Source: CAD feature listing. Evaluate the final solid. Frame: model axes, mm. Round coordinates to 2 decimals unless told otherwise and drop trailing zeros. Order: outer loops, then holes, each group sorted by start corner. A loop starts at its lowest first (then second) coordinate and runs counter-clockwise, first axis right, second up. Notation, with made-up numbers: M -30,7 L 26,7 A17 cw 26,18 Z; hole C 15.5,78 d5. An arc over 180 degrees is marked long. Use one line per item in the form item = value. Start each with the question number.
Q1. Material intervals for probe 1 along Z at (x, y) = (-15, -0.25); probe 2 along Y at (x, z) = (19, 21.5); probe 3 along X at (y, z) = (9.25, 21), sorted ascending.
Q2. Contact query for flat-ended pins moving along their axis: pin 1 (2.5 mm diameter, centred on y = 4, z = 26.5, fed in from +X); pin 2 (0.6 mm diameter, centred on x = -1, y = 11, fed in from +Z); pin 3 (0.6 mm diameter, centred on y = 11, z = 29.5, fed in from +X). Output: stop coordinate, or through.
Q3. Section A-A (x = -26). Return the cut outline in (y, z), plus the area to 3 significant figures.
Q4. Section C-C (y = 3). Return the cut outline in (x, z).
Q5. Section B-B (z = 18). Return the cut outline in (x, y).
Q6. Pull-direction query (Y, two-part tool) for faces 1 (the cylindrical face through (-30.78, 0.9, -0.44)), 2 (the flat face through (0, 6, 28.85)), 3 (the flat face through (0, 6, 20.35)), 4 (the flat face through (0, 0, 31.35)); classes: pulls with the +Y half, pulls with the -Y half, needs draft (parallel to the pull), parting line crosses it, or undercut.
Autodesk Inventor part; units mm, degrees
ref_plane "YZ Plane" through (0, 0, 0) normal (1, 0, 0) x (0, 1, 0)
ref_plane "XZ Plane" through (0, 0, 0) normal (0, 1, 0) x (-1, 0, 0)
ref_plane "XY Plane" through (0, 0, 0) normal (0, 0, 1) x (1, 0, 0)
sketch "Skizze1" plane through (0, 0, 0) normal (0, 1, 0) x (-1, 0, 0)
  line L0 (-31.35, 31.35) -> (31.35, 31.35)
  line L1 (31.35, 31.35) -> (31.35, -31.35)
  line L2 (31.35, -31.35) -> (-31.35, -31.35)
  line L3 (-31.35, -31.35) -> (-31.35, 31.35)
  line L4 (-31.35, 31.35) -> (31.35, -31.35) construction
  line L5 (31.35, 31.35) -> (-31.35, -31.35) construction
  point P0 (0, 0)
  dimension "d0" = 62.7
  dimension "d1" = 62.7
extrude "Extrusion1" add sketch "Skizze1" along normal mid plane 3
sketch "Skizze2" plane through (0, 1.5, 0) normal (0, 1, 0) x (1, 0, 0)
  line L0 (-31.35, -31.35) -> (31.35, -31.35) construction
  line L1 (0, -31.35) -> (0, 0) construction
  line L2 (4.25, -28.85) -> (-4.25, -28.85)
  line L3 (-4.25, -28.85) -> (-4.25, -20.35)
  line L4 (-4.25, -20.35) -> (4.25, -20.35)
  line L5 (4.25, -20.35) -> (4.25, -28.85)
  dimension "d6" = 2.5
  dimension "d7" = 8.5
  dimension "d9" = 4.25
  dimension "d10" = 4.25
extrude "Extrusion2" add sketch "Skizze2" along normal blind 10
sketch "Skizze3" plane through (0, 11.5, 0) normal (0, 1, 0) x (1, 0, 0)
  line L0 (-4.25, -28.85) -> (-4.25, -20.35)
  line L1 (4.25, -20.35) -> (4.25, -28.85)
  line L2 (-4.25, -28.85) -> (4.25, -28.85)
  line L3 (-4.25, -26.85) -> (-5.25, -26.85)
  line L4 (4.25, -26.85) -> (5.25, -26.85)
  line L5 (-4.25, -20.35) -> (4.25, -20.35)
  line L6 (-2.25, -20.35) -> (-2.25, -19.35)
  line L7 (-2.25, -19.35) -> (2.25, -19.35)
  line L8 (2.25, -19.35) -> (2.25, -20.35)
  line L9 (-2.25, -28.85) -> (-2.25, -29.85)
  line L10 (-2.25, -29.85) -> (2.25, -29.85)
  line L11 (2.25, -29.85) -> (2.25, -28.85)
  line L12 (5.25, -26.85) -> (5.25, -22.35)
  line L13 (5.25, -22.35) -> (4.25, -22.35)
  line L14 (-5.25, -26.85) -> (-5.25, -22.35)
  line L15 (-5.25, -22.35) -> (-4.25, -22.35)
  point P0 (0, 0)
  dimension "d18" = 1
  dimension "d19" = 1
  dimension "d21" = 1
  dimension "d22" = 1
  dimension "d23" = 2
  dimension "d24" = 2
  dimension "d25" = 2
  dimension "d26" = 2
  dimension "d27" = 2
  dimension "d28" = 2
  dimension "d29" = 2
extrude "Extrusion3" add sketch "Skizze3" against normal blind 0.5 contours L3 L14 L15 L0 | L2 L11 L10 L9 | L6 L7 L8 L5 | L1 L13 L12 L4
fillet "Rundung1" radius 2 3 edges at (-31.35, 1.5, 0) (0, 1.5, -31.35) (31.35, 1.5, 0)
properties part number "GroundV11"
Results list:
q1.probe_1 = -31.33 to 31.35
q1.probe_2 = -1.5 to 1.5
q1.probe_3 = -4.25 to 4.25
q2.pin_1 = 4.25
q2.pin_2 = 29.85
q2.pin_3 = 2.25
q3.outline = M -1.5,-31.35 L -0.5,-31.35 A2 ccw 1.5,-29.35 L 1.5,31.35 L -1.5,31.35 Z
q3.area = 187 mm2
q4.outline = M -4.25,20.35 L 4.25,20.35 L 4.25,28.85 L -4.25,28.85 Z
q5.outline = M -31.35,-1.5 L 31.35,-1.5 L 31.35,-0.5 A2 ccw 29.35,1.5 L -29.35,1.5 A2 ccw -31.35,-0.5 Z
q6.face_1 = pulls with the +Y half
q6.face_2 = undercut
q6.face_3 = undercut
q6.face_4 = needs draft
